For this review, take the finished solid that the model builds, in its own axes (mm). A direction names the side the tool comes from. Round coordinates to 2 decimals unless told otherwise and drop trailing zeros. Order: outer loops, then holes, each group sorted by start corner. A loop starts at its lowest first (then second) coordinate and runs counter-clockwise, first axis right, second up. Notation, with made-up numbers: M 77.25,77.25 L 116.25,77.25 A23 ccw 116.25,109.25 Z; hole C 20,-12.5 d8. An arc over 180 degrees is marked long. Answer as a JSON object with one key per item and string values.
Autodesk Inventor part; units mm, degrees
ref_plane "YZ Plane" through (0, 0, 0) normal (1, 0, 0) x (0, 1, 0)
ref_plane "XZ Plane" through (0, 0, 0) normal (0, 1, 0) x (-1, 0, 0)
ref_plane "XY Plane" through (0, 0, 0) normal (0, 0, 1) x (1, 0, 0)
sketch "Sketch1" plane through (0, 0, 0) normal (0, 0, 1) x (1, 0, 0)
  line L0 (-10, -3.45) -> (10, -3.45)
  line L1 (10, -3.45) -> (10, 3.45)
  line L2 (10, 3.45) -> (-10, 3.45)
  line L3 (-10, 3.45) -> (-10, -3.45)
  line L4 (-10, -3.45) -> (10, 3.45) construction
  line L5 (10, -3.45) -> (-10, 3.45) construction
  point P0 (0, 0)
  dimension "d0" = 20
  dimension "d1" = 6.9
extrude "Extrusion1" add sketch "Sketch1" along normal blind 5
sketch "Sketch2" plane through (-10, -3.45, 0) normal (0, -1, 0) x (1, 0, 0)
  line L0 (0, 0) -> (20, 0) construction
  line L1 (20, 0) -> (20, 5) construction
  line L2 (0, 5) -> (20, 5) construction
  line L3 (0, 0) -> (0, 5) construction
  line L4 (0, 2.5) -> (20, 2.5) construction
  line L5 (10, 0) -> (10, 9.5166) construction
  point P0 (5, 2.5)
  point P1 (15, 2.5)
  dimension "d4" = 5
hole "Hole1" at (-5, -3.45, 2.5) at (5, -3.45, 2.5) direction (0, 1, 0) diameter 2.459 depth 6 tip angle 118
equation "\"d1\" = front_length"
equation "\"front_length\" = 6.9"
properties part number "tap_straight_bottom" material "Aluminum 6061"
1) Add section A-A on y = 1.75. State the section outline as (x, z) points, and give its area (3 significant figures).
Geometry check:
{"outline": "M -10,0 L 10,0 L 10,5 L -10,5 Z; hole C -5,2.5 d2.46; hole C 5,2.5 d2.46", "area": "90.5 mm²"}
2) Mouldability with a two-part tool opening along Z and no side actions: class faces 3 (the cylindrical face through (-3.91, -0.41, 1.93)), 4 (the flat face through (0, 0, 5)), 5 (the flat face through (0, 0, 0)) as +Z half, -Z half, draft (parallel to the pull), parting line (faces both ways), or undercut.
Geometry check:
{"face 3": "undercut", "face 4": "+Z half", "face 5": "-Z half"}
3) Machinability: for faces 1 (the flat face through (0, -3.45, 2)), 2 (the cylindrical face through (6.09, -0.41, 1.93)), which of the approach directions +Z, -Z, +X, -X, +Y, -Y give a long, thin tool a straight path to every point of the face, cutting with its end or side? Answer none if there is none.
Geometry check:
{"face 1": "+Z, -Z, +X, -X, -Y", "face 2": "-Y"}
4) For L1, parallel to X at y = -0.1, z = 2.5; L2, parallel to Z at x = -5, y = -1.1; L3, parallel to X at y = 0.75, z = 2.05, list the stretches that pass through material, from the lowest coordinate up.
Geometry check:
{"L1": "x = -10 to -6.23, -3.77 to 3.77, 6.23 to 10", "L2": "z = 0 to 1.27, 3.73 to 5", "L3": "x = -10 to -6.14, -3.86 to 3.86, 6.14 to 10"}
